Source: CAD feature listing. Evaluate the final solid. Frame: model axes, mm. Round coordinates to 2 decimals unless told otherwise and drop trailing zeros. Write each loop counter-clockwise with the first axis right and the second up, starting at its lowest first coordinate (ties: lowest second). Pieces come first, ordered by that corner, then holes.
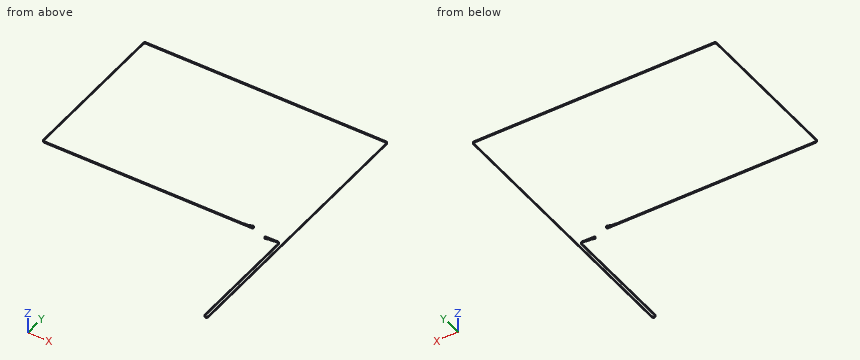
from build123d import *

# Parameters (mm, degrees)
EXTRUDE_THIN4_DEPTH = 6


with BuildPart() as part:
    # Sketch1 → Extrude-Thin4 (new body)
    with BuildSketch(Plane.XY.offset(93.86849497)):
        with BuildLine():
            Line((454.547451712, -84.747722447), (436.143146619, -85.206883154))
            ThreePointArc((436.143146619, -85.206883154), (435.325389653, -85.293870004), (434.532383495, -85.511664405))
            Line((434.532383495, -85.511664405), (424.523003293, -89.154780862))
            ThreePointArc((424.523003293, -89.154780862), (420.309165105, -86.756830797), (423.355608829, -82.985123303))
            Line((423.355608829, -82.985123303), (471.385170996, -81.786855419))
            ThreePointArc((471.385170996, -81.786855419), (476.52965679, -83.807458497), (478.672495941, -88.902241246))
            Line((478.672495941, -88.902241246), (478.192503637, -538.093193208))
            ThreePointArc((478.192503637, -538.093193208), (484.559857096, -544.469999452), (490.932499818, -538.098479016))
            Line((490.932499818, -538.098479016), (490.672499826, 550.801458903))
            ThreePointArc((490.672499826, 550.801458903), (488.882406602, 555.120938203), (484.5625, 556.91))
            Line((484.5625, 556.91), (-471.5625, 556.91))
            ThreePointArc((-471.5625, 556.91), (-475.882922433, 555.120422433), (-477.6725, 550.8))
            Line((-477.6725, 550.8), (-477.6725, -58.894643712))
            ThreePointArc((-477.6725, -58.894643712), (-475.882402145, -63.215586371), (-471.56102849, -65.004643535))
            Line((-471.56102849, -65.004643535), (356.760717872, -64.80515362))
            ThreePointArc((356.760717872, -64.80515362), (359.892804832, -61.071108191), (355.671900131, -58.634506563))
            Line((355.671900131, -58.634506563), (340.245690102, -64.249187841))
            ThreePointArc((340.245690102, -64.249187841), (339.390962941, -64.478266451), (338.509451222, -64.55554918))
            Line((338.509451222, -64.55554918), (325.647451712, -64.558646816))
            Line((325.647451712, -64.558646816), (325.647210875, -63.558646845))
            Line((325.647210875, -63.558646845), (338.509210386, -63.555549209))
            ThreePointArc((338.509210386, -63.555549209), (339.217196175, -63.493479616), (339.903669959, -63.30949522))
            Line((339.903669959, -63.30949522), (355.329879987, -57.694813942))
            ThreePointArc((355.329879987, -57.694813942), (360.877591668, -60.897341426), (356.760958708, -65.805153591))
            Line((356.760958708, -65.805153591), (-471.560787654, -66.004643506))
            ThreePointArc((-471.560787654, -66.004643506), (-476.589423772, -63.922778296), (-478.6725, -58.894643712))
            Line((-478.6725, -58.894643712), (-478.6725, 550.8))
            ThreePointArc((-478.6725, 550.8), (-476.590029214, 555.827529214), (-471.5625, 557.91))
            Line((-471.5625, 557.91), (484.5625, 557.91))
            ThreePointArc((484.5625, 557.91), (489.589428959, 555.828129398), (491.672499797, 550.801697677))
            Line((491.672499797, 550.801697677), (491.93249979, -538.098240242))
            ThreePointArc((491.93249979, -538.098240242), (484.559442197, -545.469999366), (477.192504208, -538.092124638))
            Line((477.192504208, -538.092124638), (477.672496512, -88.901172676))
            ThreePointArc((477.672496512, -88.901172676), (475.831041208, -84.522955714), (471.410111784, -82.786544349))
            Line((471.410111784, -82.786544349), (423.380549617, -83.984812234))
            ThreePointArc((423.380549617, -83.984812234), (421.29173064, -86.570914228), (424.180983149, -88.215088242))
            Line((424.180983149, -88.215088242), (434.190363351, -84.571971785))
            ThreePointArc((434.190363351, -84.571971785), (435.139473084, -84.31130447), (436.11820583, -84.207194224))
            Line((436.11820583, -84.207194224), (454.522510923, -83.748033516))
            Line((454.522510923, -83.748033516), (454.547451712, -84.747722447))
        make_face()
    extrude(amount=EXTRUDE_THIN4_DEPTH)


solid = part.part
1) Contact query for flat-ended pins moving along their axis: P1, Ø5.5, axis at x = 356.76, y = -61.62, coming from the +Z side; P2, Ø3, axis at x = 333, z = 96, coming from the -Y side; P3, Ø5.5, axis at x = 423.43, y = -86.17, coming from the +Z side; P4, Ø1.5, axis at x = -223, z = 96, coming from the -Y side. Output: stop coordinate, or through.
Taken from the geometry:
P1: passes through
P2: stops at y = -65.81
P3: stops at z = 99.87
P4: stops at y = -65.94
2) Material intervals for line 1 (Y direction, x = 442.5, z = 97.6); line 2 (Y direction, x = -240.5, z = 98.8); line 3 (X direction, y = -364, z = 97.6), sorted ascending.
Taken from the geometry:
line 1: y = -85.05 to -84.05, -83.51 to -82.51, 556.91 to 557.91
line 2: y = -65.95 to -64.95, 556.91 to 557.91
line 3: x = 477.38 to 478.38, 490.89 to 491.89
3) Section query B-B on x = -327. Return the cut outline in (y, z).
Taken from the geometry:
outline: (-65.97, 93.87) - (-64.97, 93.87) - (-64.97, 99.87) - (-65.97, 99.87) - close; (556.91, 93.87) - (557.91, 93.87) - (557.91, 99.87) - (556.91, 99.87) - close
4) Section query A-A on y = 342.5. Return the cut outline in (x, z), then the cut area to 3 significant figures.
Taken from the geometry:
outline: (-478.67, 93.87) - (-477.67, 93.87) - (-477.67, 99.87) - (-478.67, 99.87) - close; (490.72, 93.87) - (491.72, 93.87) - (491.72, 99.87) - (490.72, 99.87) - close
area: 12.0 mm2
